from build123d import *

# Parameters (mm, degrees)
SKETCH2_W          = 6
SKETCH2_H          = 3.873628034
CUT_EXTRUDE1_DEPTH = 70.670653793
CIRPATTERN1_COUNT  = 3
SKETCH4_W          = 2.5
SKETCH4_H          = 43
CIRPATTERN2_COUNT  = 2
CIRPATTERN2_ANGLE  = 90
FILLET1_R          = 0.762


with BuildPart() as part:
    # Sketch1 → Revolve1 (revolve)
    with BuildSketch(Plane.XY, mode=Mode.PRIVATE) as revolve1_sk:
        Polygon((0, 34.9501), (0, 43), (34, 43), (34, 30.125), (28, 30.125), (28, 34.6881), (17, 34.6881), (17, 34.1881), (0.762, 34.1881), align=None)
    revolve(revolve1_sk.sketch.rotate(Axis((0, 0, 0), (-1, 0, 0)), 90), axis=Axis((0, 0, 0), (-1, 0, 0)))

    # Sketch2 → Cut-Extrude1 (cut, through all)
    with BuildSketch(Plane.ZY):
        with Locations((0, 42.052814017)):
            Rectangle(SKETCH2_W, SKETCH2_H)
    cut_extrude1 = extrude(amount=-CUT_EXTRUDE1_DEPTH, mode=Mode.SUBTRACT)

    # CirPattern1: Cut-Extrude1 ×3 about axis
    cirpattern1_axis = Axis((0, 0, 0), (1, 0, 0))
    for i in range(1, CIRPATTERN1_COUNT):
        add(cut_extrude1.rotate(cirpattern1_axis, i * 360 / CIRPATTERN1_COUNT), mode=Mode.SUBTRACT)

    # Sketch4 → M6 Tapped Hole1 (revolve, cut)
    with BuildSketch(Plane(origin=(21, 0, 0), x_dir=(0, 0, 1), z_dir=(1, 0, 0))):
        with Locations((1.25, 21.5)):
            Rectangle(SKETCH4_W, SKETCH4_H)
    m6_tapped_hole1 = revolve(axis=Axis((21, 6.35, 0), (0, -1, 0)), mode=Mode.SUBTRACT)

    # CirPattern2: M6 Tapped Hole1 ×2 about axis
    cirpattern2_axis = Axis((0, 0, 0), (1, 0, 0))
    for i in range(1, CIRPATTERN2_COUNT):
        add(m6_tapped_hole1.rotate(cirpattern2_axis, i * CIRPATTERN2_ANGLE / (CIRPATTERN2_COUNT - 1)), mode=Mode.SUBTRACT)

    # Fillet1
    fillet1_edges = [part.edges().sort_by_distance(p)[0] for p in [
        (28, 0, 34.6881),
    ]]
    fillet(fillet1_edges, radius=FILLET1_R)


solid = part.part
Build history of the part. All positions in model axes, mm. A direction names the side the tool comes from. Round coordinates to 2 decimals unless told otherwise and drop trailing zeros. Order: outer loops, then holes, each group sorted by start corner. A loop starts at its lowest first (then second) coordinate and runs counter-clockwise, first axis right, second up. Notation, with made-up numbers: M 6.5,84.5 L 61.5,84.5 A37 cw 61.5,123.5 Z; hole C 61,28 d1. An arc over 180 degrees is marked long. Use CSV: the item, a comma, the result in double quotes. Start each with the question number.
(1) Cut at D-D on x = 21. List the corners of the cut face in (y, z).
(2) Drill centre lines: probe 1 along X at (y, z) = (-38, 0); probe 2 along Z at (x, y) = (23.5, 0.5); probe 3 along Y at (x, z) = (4, 0). Where is each one in solid material? Low to high.
(3) Cut at B-B on z = 0. List the corners of the cut face in (x, y) (3 decimals).
(4) Cut at C-C on x = 3.5. List the corners of the cut face in (y, z).
(5) Flat gauge pins, fed straight in: P1, Ø2, axis at x = 15.5, z = 31.5, coming from the -Y side; P2, Ø1, axis at x = 21, y = 0, coming from the -Z side; P3, Ø1.8, axis at x = 15.5, z = 0, coming from the +Y side. Where does each tip first touch, or does it go through?
(6) Tool access for faces 5 (the face through (17, 41, 3)), 6 (the face through (18.52, 0.33, -38.86)), 7 (the face through (16.762, -20.022, 34.762)), 8 (the face through (16.762, -18.145, 37.428)), 9 (the face through (17, 23, -25.5)): list every direction of +Z, -Z, +X, -X, +Y, -Y with a clear straight run to the whole face (end or side of a thin tool).
(7) Cut at A-A on y = 0. List the corners of the cut face in (x, z) (3 decimals), then the cut area to 3 significant figures.
(8) Mould opens along Z. For faces 1 (the face through (17.24, 22.01, -36.94)), 2 (the face through (34, 9, 29)), 3 (the face through (8.767, 33.375, 7.411)), 4 (the face through (16.76, -23.34, 34.43)) say: +Z half, -Z half, draft (parallel to the pull), parting line (faces both ways), or undercut.
Findings:
1,outline,"M -42.93,-2.5 A43 ccw -24.05,-35.65 L -22.66,-33.24 L -17.46,-36.24 L -18.85,-38.65 A43 ccw -2.5,-42.93 L -2.5,-34.6 A34.69 cw -34.6,-2.5 Z; M -42.93,2.5 L -34.6,2.5 A34.69 cw long 2.5,-34.6 L 2.5,-42.93 A43 ccw 42.9,-3 L 40.12,-3 L 40.12,3 L 42.9,3 A43 ccw -18.85,38.65 L -17.46,36.24 L -22.66,33.24 L -24.05,35.65 A43 ccw Z"
2,probe 1,"x = 0 to 18.5, 23.5 to 34"
2,probe 2,"z = -43 to -34.68, 34.68 to 43"
2,probe 3,"y = -43 to -34.19, 34.19 to 40.12"
3,outline,"M 0,-43 L 18.5,-43 L 18.5,-34.688 L 17,-34.688 L 17,-34.188 L 0.762,-34.188 L 0,-34.95 Z; M 0,34.95 L 0.762,34.188 L 17,34.188 L 17,34.688 L 27.238,34.688 A0.762 cw 28,33.926 L 28,30.125 L 34,30.125 L 34,40.116 L 0,40.116 Z; M 23.5,-43 L 34,-43 L 34,-30.125 L 28,-30.125 L 28,-33.926 A0.762 cw 27.238,-34.688 L 23.5,-34.688 Z"
4,outline,"M -24.05,-35.65 L -22.66,-33.24 L -17.46,-36.24 L -18.85,-38.65 A43 ccw 42.9,-3 L 40.12,-3 L 40.12,3 L 42.9,3 A43 ccw -18.85,38.65 L -17.46,36.24 L -22.66,33.24 L -24.05,35.65 A43 ccw Z; hole C 0,0 d68.38"
5,P1,"stops at y = -30.31"
5,P2,"stops at z = 34.68"
5,P3,"stops at y = 40.12"
6,face 5,"+X, -X, +Y"
6,face 6,"-Z"
6,face 7,"+X, -X"
6,face 8,"+X, -X, -Y"
6,face 9,"none"
7,outline,"M 0,-43 L 18.5,-43 L 18.5,-34.688 L 17,-34.688 L 17,-34.188 L 0.762,-34.188 L 0,-34.95 Z; M 0,34.95 L 0.762,34.188 L 17,34.188 L 17,34.688 L 27.238,34.688 A0.762 cw 28,33.926 L 28,30.125 L 34,30.125 L 34,43 L 0,43 Z; M 23.5,-43 L 34,-43 L 34,-30.125 L 28,-30.125 L 28,-33.926 A0.762 cw 27.238,-34.688 L 23.5,-34.688 Z"
7,area,"595 mm^2"
8,face 1,"-Z half"
8,face 2,"draft"
8,face 3,"undercut"
8,face 4,"+Z half"
